Could you check a few things on this model? Use its own coordinates, in mm. A direction names the side the tool comes from. Round coordinates to 2 decimals unless told otherwise and drop trailing zeros. Order: outer loops, then holes, each group sorted by start corner. A loop starts at its lowest first (then second) coordinate and runs counter-clockwise, first axis right, second up. Notation, with made-up numbers: M 39,25 L 62,25 A34 ccw 62,56 Z; hole C -14.5,34 d6. An arc over 180 degrees is marked long. Write each question's results on one line, items separated by ' | '. Start each with the question number.
1. Please list where these lines run through material, in increasing order: L1, parallel to Y at x = 0, z = 6.5; L2, parallel to Y at x = -5, z = -16; L3, parallel to Z at x = -1, y = 49.
2. Suppose I cut it at D-D on x = -9. Write out the boundary of the cut face in (y, z).
3. Suppose I cut it at B-B on z = 0. Write out the boundary of the cut face in (x, y), and give its area (3 significant figures).
4. Suppose I cut it at C-C on y = 107. Write out the boundary of the cut face in (x, z), and give its area (3 significant figures).
5. For faces 1 (the cylindrical face through (5.362, 100.74, -12.932)), 2 (the flat face through (0, 192, 0)), which set-ups out of +Z, -Z, +X, -X, +Y, -Y let a thin tool reach every point of the face, with its end or its side?
6. Suppose I cut it at A-A on x = 0. Write out the boundary of the cut face in (y, z), and give its area (3 significant figures).
7. We'd pull the mould along Y, two halves only. Please class faces 3 (the cylindrical face through (7.509, 5.916, 23.846)), 4 (the flat face through (-11, 12, 11)), 5 (the cylindrical face through (-0.751, 185.385, 0.196)), 6 (the flat face through (0, 0, 0)): released by +Y, released by -Y, zero draft, split by the parting line, or undercut.
8. I'm going to push flat-ended pins straight in: pin 1 (10 mm diameter, centred on y = 88, z = 14, fed in from +X); pin 2 (5 mm diameter, centred on x = 15, y = 67, fed in from +Z); pin 3 (10 mm diameter, centred on x = 8, y = 20, fed in from -Z); pin 4 (2 mm diameter, centred on y = 64.5, z = 15.5, fed in from +X). Where does each tip first touch, or does it pass through?
from build123d import *

# Parameters (mm, degrees)
SKETCH1_R           = 25
BOSS_EXTRUDE1_DEPTH = 12
SKETCH2_R           = 14
BOSS_EXTRUDE2_DEPTH = 180
SKETCH3_R           = 2.5
CUT_EXTRUDE1_DEPTH  = 90


with BuildPart() as part:
    # Sketch1 → Boss-Extrude1 (new body)
    with BuildSketch(Plane(origin=(0, 0, 0), x_dir=(1, 0, 0), z_dir=(0, 1, 0))):
        with Locations(Location((0, 0, 0), (0, 0, 270))):
            Circle(SKETCH1_R)
    extrude(amount=BOSS_EXTRUDE1_DEPTH)

    # Sketch2 → Boss-Extrude2 (add)
    with BuildSketch(Plane(origin=(0, 12, 0), x_dir=(1, 0, 0), z_dir=(0, 1, 0))):
        with Locations(Location((0, 0, 0), (0, 0, 90))):
            Circle(SKETCH2_R)
    extrude(amount=BOSS_EXTRUDE2_DEPTH)

    # Sketch3 → Cut-Extrude1 (cut, symmetric)
    with BuildSketch(Plane.XY):
        with Locations(Location((0, 183, 0), (0, 0, 90.000000007))):
            Circle(SKETCH3_R)
    extrude(amount=CUT_EXTRUDE1_DEPTH, both=True, mode=Mode.SUBTRACT)


solid = part.part
Filled sheet:
1) L1: y = 0 to 180.5, 185.5 to 192 | L2: y = 0 to 12 | L3: z = -13.96 to 13.96
2) outline: M 0,-23.32 L 12,-23.32 L 12,-10.72 L 192,-10.72 L 192,10.72 L 12,10.72 L 12,23.32 L 0,23.32 Z
3) outline: M -25,0 L 25,0 L 25,12 L 14,12 L 14,192 L -14,192 L -14,12 L -25,12 Z; hole C 0,183 d5 | area: 5,620 mm^2
4) outline: C 0,0 d28 | area: 616 mm^2
5) face 1: +Y | face 2: +Z, -Z, +X, -X, +Y
6) outline: M 0,-25 L 12,-25 L 12,-14 L 180.5,-14 L 180.5,14 L 12,14 L 12,25 L 0,25 Z; M 185.5,-14 L 192,-14 L 192,14 L 185.5,14 Z | area: 5,500 mm^2
7) face 3: zero draft | face 4: released by +Y | face 5: undercut | face 6: released by -Y
8) pin 1: stops at x = 10.72 | pin 2: stops at z = 6.3 | pin 3: stops at z = -13.67 | pin 4: passes through
